Geometry check sheet. Reference: the model listing, model coordinates, mm. Face numbers are marked on the shaded views. A direction names the side the tool comes from. Round coordinates to 2 decimals unless told otherwise and drop trailing zeros. Write each loop counter-clockwise with the first axis right and the second up, starting at its lowest first coordinate (ties: lowest second). Pieces come first, ordered by that corner, then holes. Notation, with made-up numbers: (58, -39) - (100, -39) arc R16 ccw to (100, -16) - close; hole circle Ø7 at (65.5, 65). An arc over 180 degrees is marked (long way). Return JSON: item names as keys, results as strings.
```python
from build123d import *

# Parameters (mm, degrees)
SKETCH1_R           = 6.575
SKETCH1_R_2         = 1
BOSS_EXTRUDE1_DEPTH = 2
SKETCH2_R           = 5.85
BOSS_EXTRUDE2_DEPTH = 1
SKETCH3_R           = 4.95
BOSS_EXTRUDE3_DEPTH = 0.5
BOSS_EXTRUDE4_DEPTH = 3.4
SKETCH6_R           = 1.1
CUT_EXTRUDE1_DEPTH  = 4
BOSS_EXTRUDE5_DEPTH = 0.4
SKETCH8_W           = 10.55
SKETCH8_H           = 8.790176683
CUT_EXTRUDE2_DEPTH  = 0.1


with BuildPart() as part:
    # Sketch1 → Boss-Extrude1 (new body)
    with BuildSketch(Plane(origin=(0, 0, 0), x_dir=(1, 0, 0), z_dir=(0, 1, 0))):
        with Locations((0, -7.9)):
            Circle(SKETCH1_R)
        with BuildLine():
            Line((-2.85, 10), (-5.575, 10))
            ThreePointArc((-5.575, 10), (-4.867893219, 9.707106781), (-4.575, 9))
            ThreePointArc((-4.575, 9), (-5.574999999, 8), (-6.575, 8.999999999))
            Line((-6.575, 8.999999999), (-6.575, -7.9))
            ThreePointArc((-6.575, -7.9), (0, -1.325), (6.575, -7.9))
            Line((6.575, -7.9), (6.575, 9))
            ThreePointArc((6.575, 9), (4.867893224, 8.292893214), (5.574999986, 10))
            Line((5.574999986, 10), (2.85, 10))
            ThreePointArc((2.85, 10), (0, 7.15), (-2.85, 10))
        make_face()
        with Locations((-5.575, 9)):
            Circle(SKETCH1_R_2)
        with BuildLine():
            ThreePointArc((2.85, 10), (0, 12.85), (-2.85, 10))
            Line((-2.85, 10), (2.85, 10))
        make_face()
        with BuildLine():
            Line((2.85, 10), (-2.85, 10))
            ThreePointArc((-2.85, 10), (0, 7.15), (2.85, 10))
        make_face()
        with Locations((5.575, 9)):
            Circle(SKETCH1_R_2)
    extrude(amount=BOSS_EXTRUDE1_DEPTH)

    # Sketch2 → Boss-Extrude2 (add)
    with BuildSketch(Plane(origin=(0, 2, 0), x_dir=(-1, 0, 0), z_dir=(0, 1, 0))):
        with Locations((0, 7.9)):
            Circle(SKETCH2_R)
    extrude(amount=BOSS_EXTRUDE2_DEPTH)

    # Sketch3 → Boss-Extrude3 (add)
    with BuildSketch(Plane(origin=(0, 3, 0), x_dir=(-1, 0, 0), z_dir=(0, 1, 0))):
        with Locations((0, 7.9)):
            Circle(SKETCH3_R)
    extrude(amount=BOSS_EXTRUDE3_DEPTH)

    # Sketch4 → Boss-Extrude4 (add)
    with BuildSketch(Plane(origin=(0, 3.5, 0), x_dir=(-1, 0, 0), z_dir=(0, 1, 0))):
        Polygon((2.736417755, 7.190894071), (2.518440958, 7.568440958), (2.831329546, 7.881329546), (2.828587818, 7.921412182), (2.518440958, 8.231559042), (2.741390732, 8.617719379), (2.729517437, 8.651127629), (2.346813369, 8.872081926), (2.463209043, 9.306476495), (2.445926072, 9.330960886), (2.015254326, 9.446359032), (2.015254326, 9.900296057), (1.996868143, 9.915254326), (1.546359032, 9.915254326), (1.427678707, 10.35817533), (1.412422166, 10.36480218), (0.972081926, 10.246813369), (0.740314632, 10.648246096), (0.731654815, 10.64943636), (0.331559042, 10.418440958), (0, 10.75), (-0.331559042, 10.418440958), (-0.731654815, 10.64943636), (-0.740314632, 10.648246096), (-0.972081926, 10.246813369), (-1.412422166, 10.36480218), (-1.427678707, 10.35817533), (-1.546359032, 9.915254326), (-1.996868143, 9.915254326), (-2.015254326, 9.900296057), (-2.015254326, 9.446359032), (-2.445926072, 9.330960886), (-2.463209043, 9.306476495), (-2.346813369, 8.872081926), (-2.729517437, 8.651127629), (-2.741390732, 8.617719379), (-2.518440958, 8.231559042), (-2.828587818, 7.921412182), (-2.831329546, 7.881329546), (-2.518440958, 7.568440958), (-2.736417755, 7.190894071), (-2.727435802, 7.147670539), (-2.346813369, 6.927918074), (-2.459115706, 6.508800044), (-2.437318125, 6.466732622), (-2.015254326, 6.353640968), (-2.015254326, 5.921202275), (-1.981206238, 5.884745674), (-1.546359032, 5.884745674), (-1.434668452, 5.467910755), (-1.390523426, 5.441065569), (-0.972081926, 5.553186631), (-0.756489757, 5.179770042), (-0.705710775, 5.165542438), (-0.331559042, 5.381559042), (-0.026545054, 5.076545054), (0.026545054, 5.076545054), (0.331559042, 5.381559042), (0.705710775, 5.165542438), (0.756489757, 5.179770042), (0.972081926, 5.553186631), (1.390523426, 5.441065569), (1.434668452, 5.467910755), (1.546359032, 5.884745674), (1.981206238, 5.884745674), (2.015254326, 5.921202275), (2.015254326, 6.353640968), (2.437318125, 6.466732622), (2.459115706, 6.508800044), (2.346813369, 6.927918074), (2.727435802, 7.147670539), align=None)
    extrude(amount=BOSS_EXTRUDE4_DEPTH)

    # Sketch5 → Cut-Revolve1 (revolve, cut)
    with BuildSketch(Plane(origin=(0, 0, 0), x_dir=(0, 0, -1), z_dir=(1, 0, 0))):
        Polygon((-5.867221225, 7.3), (-4.517199782, 7.3), (-4.517199782, 5.949978558), align=None)
    revolve(axis=Axis((0, 8.077813164, 7.836091173), (0, -1, 0)), mode=Mode.SUBTRACT)

    # Sketch6 → Cut-Extrude1 (cut)
    with BuildSketch(Plane(origin=(0, 6.9, 0), x_dir=(-1, 0, 0), z_dir=(0, 1, 0))):
        with Locations((0, 7.836091173)):
            Circle(SKETCH6_R)
    extrude(amount=-CUT_EXTRUDE1_DEPTH, mode=Mode.SUBTRACT)

    # Sketch7 → Boss-Extrude5 (add)
    with BuildSketch(Plane(origin=(0, 2, 0), x_dir=(-1, 0, 0), z_dir=(0, 1, 0))):
        with BuildLine():
            Line((2.532291452, -9.7), (5.575, -9.7))
            ThreePointArc((5.575, -9.7), (6.069974747, -9.494974747), (6.275, -9))
            Line((6.275, -9), (6.275, 1.090176683))
            Line((6.275, 1.090176683), (-6.275, 1.090176683))
            Line((-6.275, 1.090176683), (-6.275, -1.654552581))
            Line((-6.275, -1.654552581), (-6.275, -9))
            ThreePointArc((-6.275, -9), (-6.069974747, -9.494974747), (-5.575, -9.7))
            Line((-5.575, -9.7), (-2.532291452, -9.7))
            ThreePointArc((-2.532291452, -9.7), (0, -12.55), (2.532291452, -9.7))
        make_face()
    extrude(amount=BOSS_EXTRUDE5_DEPTH)

    # Sketch8 → Cut-Extrude2 (cut)
    with BuildSketch(Plane(origin=(0, 2.4, 0), x_dir=(-1, 0, 0), z_dir=(0, 1, 0))):
        with Locations((0, -4.304911659)):
            Rectangle(SKETCH8_W, SKETCH8_H)
    extrude(amount=-CUT_EXTRUDE2_DEPTH, mode=Mode.SUBTRACT)


solid = part.part
```
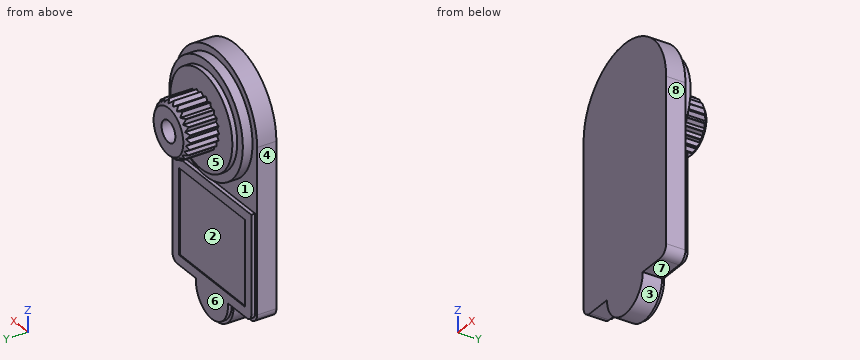
(1) Access from +Z, -Z, +X, -X, +Y, -Y to the whole of each face (thin tool, end or side, straight path). Record for the marked faces 5, 6, 7 and 8.
Response values:
{"face 5": "+Y", "face 6": "-Z, +X, -X, +Y", "face 7": "-Z, +X, +Y, -Y", "face 8": "+Z, -Z, +X, +Y, -Y"}
(2) Section check A-A, the plane z = -1. Enter the section's corners in (x, y) (3 decimals).
Response values:
{"outline": "(-6.575, 0) - (6.575, 0) - (6.575, 2) - (6.275, 2) - (6.275, 2.4) - (5.275, 2.4) - (5.275, 2.3) - (-5.275, 2.3) - (-5.275, 2.4) - (-6.275, 2.4) - (-6.275, 2) - (-6.575, 2) - close"}
(3) Section check B-B, the plane x = -3.5. Enter the section's corners in (y, z), plus the area to 3 significant figures.
Response values:
{"outline": "(0, -10) - (2, -10) - (2, -9.7) - (2.4, -9.7) - (2.4, -8.7) - (2.3, -8.7) - (2.3, 0.09) - (2.4, 0.09) - (2.4, 1.09) - (2, 1.09) - (2, 3.21) - (3, 3.21) - (3, 4.4) - (3.5, 4.4) - (3.5, 11.4) - (3, 11.4) - (3, 12.59) - (2, 12.59) - (2, 13.47) - (0, 13.47) - close", "area": "63.2 mm^2"}
(4) Gauge pin test, flat ends, axial feed: pin 1 (1.6 mm diameter, centred on x = -4.5, y = 1.5, fed in from -Z); pin 2 (1.5 mm diameter, centred on y = 1, z = 11, fed in from -X); pin 3 (6.5 mm diameter, centred on x = 2.5, z = 0.5, fed in from +Y). Record the tip position at first contact, or that the pin passes through.
Response values:
{"pin 1": "stops at z = -10", "pin 2": "stops at x = -6.14", "pin 3": "stops at y = 3.5"}
(5) Release check for a two-part mould opening along Z. For the marked faces 1, 2, 3 and 4 record: pulls with the +Z half, pulls with the -Z half, needs draft (parallel to the pull), parting line crosses it, or undercut.
Response values:
{"face 1": "undercut", "face 2": "undercut", "face 3": "pulls with the -Z half", "face 4": "needs draft"}
(6) Section check C-C, the plane z = 12.5. Enter the section's corners in (x, y).
Response values:
{"outline": "(-4.7, 0) - (4.7, 0) - (4.7, 2) - (3.61, 2) - (3.61, 3) - (1.83, 3) - (1.83, 3.5) - (-1.83, 3.5) - (-1.83, 3) - (-3.61, 3) - (-3.61, 2) - (-4.7, 2) - close"}
(7) Material ranges on line 1 along Y through (x, z) = (0.25, 4.75); line 2 along Y through (x, z) = (-0.25, -5.75); line 3 along Z through (x, y) = (-1.75, 6.5), recorded low to high. Write a range as [from, to].
Response values:
{"line 1": "y = [0, 3.5]", "line 2": "y = [0, 2.3]", "line 3": "z = [5.88, 9.92]"}
